```python
from build123d import *

# Parameters (mm, degrees)
SKETCH1_W           = 25.4
SKETCH1_H           = 25.4
BOSS_EXTRUDE1_DEPTH = 149.225
FILLET1_R           = 0.254
CUT_EXTRUDE1_DEPTH  = 38.1
SKETCH4_W           = 22.098
SKETCH4_H           = 22.098
CUT_EXTRUDE4_DEPTH  = 685.8
CUT_EXTRUDE5_DEPTH  = 685.8


with BuildPart() as part:
    # Sketch1 → Boss-Extrude1 (new, symmetric)
    with BuildSketch(Plane.XY):
        Rectangle(SKETCH1_W, SKETCH1_H)
    extrude(amount=BOSS_EXTRUDE1_DEPTH, both=True)

    # Fillet1
    fillet1_edges = [part.edges().sort_by_distance(p)[0] for p in [
        (-12.7, 12.7, 0),
        (-12.7, -12.7, 0),
        (12.7, -12.7, 0),
        (12.7, 12.7, 0),
    ]]
    fillet(fillet1_edges, radius=FILLET1_R)

    # Sketch2 → Cut-Extrude1 (cut)
    with BuildSketch(Plane.XZ.offset(12.7)):
        Polygon((-12.7, 149.225), (12.7, 136.283053583), (12.7, 149.225), align=None)
    extrude(amount=-CUT_EXTRUDE1_DEPTH, mode=Mode.SUBTRACT)

    # Sketch4 → Cut-Extrude4 (cut)
    with BuildSketch(Plane(origin=(0, 0, -149.225), x_dir=(-1, 0, 0), z_dir=(0, 0, -1))):
        Rectangle(SKETCH4_W, SKETCH4_H)
    extrude(amount=-CUT_EXTRUDE4_DEPTH, mode=Mode.SUBTRACT)

    # Sketch5 → Cut-Extrude5 (cut)
    with BuildSketch(Plane.XZ.offset(12.7)):
        Polygon((-12.7, -136.283053583), (-12.7, -149.225), (12.7, -149.225), align=None)
    extrude(amount=-CUT_EXTRUDE5_DEPTH, mode=Mode.SUBTRACT)


solid = part.part
```
Source: CAD feature listing. Evaluate the final solid. Frame: model axes, mm. A direction names the side the tool comes from. Give positions to 0.01 mm unless a question says otherwise; leave off trailing zeros. Write each loop counter-clockwise with the first axis right and the second up, starting at its lowest first coordinate (ties: lowest second). Pieces come first, ordered by that corner, then holes.
1. Section query B-B (z = -22.5). Return the cut outline in (x, y), then the cut area to 3 significant figures.
2. Access query for faces 4 (the face through (-11.049, 0, 4)), 5 (the face through (0.178, -11.467, -142.845)). Directions: +Z, -Z, +X, -X, +Y, -Y. A direction counts if a zero-diameter tool reaches every point of the face in a straight line with its end or side. Return the directions, or none.
3. First-contact query: pin 1 (12 mm diameter, centred on x = 4, y = 8.5, fed in from +Z); pin 2 (12 mm diameter, centred on x = -1, y = 4, fed in from -Z); pin 3 (12 mm diameter, centred on x = 9, y = -5.5, fed in from +Z). Flat tips, straight axial feed; report the tip coordinate or a pass-through.
4. Pull-direction query (X, two-part tool) for faces 1 (the face through (0, 12.7, 2)), 2 (the face through (12.7, 0, -4)), 3 (the face through (11.049, 0, -8)); classes: +X half, -X half, draft (parallel to the pull), parting line (faces both ways), or undercut.
5. Section query A-A (y = -6.75). Return the cut outline in (x, z) (3 decimals).
6. Material intervals for line 1 along X through (y, z) = (-6.25, 58), sorted ascending.
7. Section query C-C (x = 2). Return the cut outline in (y, z), then the cut area to 3 significant figures.
Output values:
1. outline: (-12.7, -12.45) arc R0.25 ccw to (-12.45, -12.7) - (12.45, -12.7) arc R0.25 ccw to (12.7, -12.45) - (12.7, 12.45) arc R0.25 ccw to (12.45, 12.7) - (-12.45, 12.7) arc R0.25 ccw to (-12.7, 12.45) - close; hole (-11.05, -11.05) - (11.05, -11.05) - (11.05, 11.05) - (-11.05, 11.05) - close
1. area: 157 mm2
2. face 4: +Z, -Z
2. face 5: -Z, -X, +Y, -Y
3. pin 1: stops at z = 143.48
3. pin 2: passes through
3. pin 3: stops at z = 139.33
4. face 1: draft
4. face 2: +X half
4. face 3: undercut
5. outline: (-12.7, -136.283) - (-11.049, -137.124) - (-11.049, 148.384) - (-12.7, 149.225) - close; (11.049, -148.384) - (12.7, -149.225) - (12.7, 136.283) - (11.049, 137.124) - close
6. line 1: x = -12.7 to -11.05, 11.05 to 12.7
7. outline: (-12.7, -143.77) - (-11.05, -143.77) - (-11.05, 141.73) - (-12.7, 141.73) - close; (11.05, -143.77) - (12.7, -143.77) - (12.7, 141.73) - (11.05, 141.73) - close
7. area: 943 mm2
